Source: CAD feature listing. Evaluate the final solid. Frame: model axes, mm. A direction names the side the tool comes from. Round coordinates to 2 decimals unless told otherwise and drop trailing zeros. Order: outer loops, then holes, each group sorted by start corner. A loop starts at its lowest first (then second) coordinate and runs counter-clockwise, first axis right, second up. Notation, with made-up numbers: (-17, 53.5) -> (36, 53.5) arc R29 cw to (36, 79.5) -> close; hole circle Ø10 at (39, 8). An arc over 180 degrees is marked (long way). Answer as CSV lines item,"result".
from build123d import *

# Parameters (mm, degrees)
SKETCH_1_W           = 2
SKETCH_1_H           = 2
EXTRUDE_1_DEPTH      = 3
EXTRUDE_2_DEPTH      = 3.25
EXTRUDE_2_DEPTH_BACK = 5.25
SKETCH_2_R           = 1.35
EXTRUDE_5_DEPTH      = 1
EXTRUDE_START        = -1
EXTRUDE_6_DEPTH      = 1
EXTRUDE_7_DEPTH      = 10
EXTRUDE_7_DEPTH_BACK = 10


with BuildPart() as part:
    # 草图1 → 凸台-拉伸1 (new body)
    with BuildSketch(Plane.XY):
        Rectangle(SKETCH_1_W, SKETCH_1_H)
    extrude(amount=EXTRUDE_1_DEPTH)

    # 草图2 → 凸台-拉伸2 (add, two sides: drawn at the far end of the back side and taken through both)
    with BuildSketch(Plane(origin=(0, 1, 0), x_dir=(1, 0, 0), z_dir=(0, 1, 0)).offset(-EXTRUDE_2_DEPTH_BACK)):
        with Locations(Location((0, -4, 0), (0, 0, 270))):
            Circle(SKETCH_2_R)
    extrude(amount=EXTRUDE_2_DEPTH + EXTRUDE_2_DEPTH_BACK)

    # 草图6 → 凸台-拉伸5 (add)
    with BuildSketch(Plane(origin=(0, -2.75, 0), x_dir=(-1, 0, 0), z_dir=(0, -1, 0))):
        with BuildLine():
            Line((-1.75, -4), (1.75, -4))
            ThreePointArc((1.75, -4), (0, -2.25), (-1.75, -4))
        make_face()
    extrude(amount=-EXTRUDE_5_DEPTH)

    # 草图7 → 凸台-拉伸6 (add)
    with BuildSketch(Plane(origin=(0, 2.75, 0), x_dir=(1, 0, 0), z_dir=(0, 1, 0)).offset(EXTRUDE_START)):
        with BuildLine():
            Line((1.75, -4), (-1.75, -4))
            ThreePointArc((-1.75, -4), (0, -2.25), (1.75, -4))
        make_face()
    extrude(amount=EXTRUDE_6_DEPTH)

    # 草图12 → 凸台-拉伸7 (add, two sides: drawn at the far end of the back side and taken through both)
    with BuildSketch(Plane(origin=(0, 0, 0), x_dir=(1, 0, 0), z_dir=(0, 1, 0)).offset(-EXTRUDE_7_DEPTH_BACK)):
        Polygon((10, 0), (-10, 0), (-14, 6.92820323), (-12.267949192, 7.92820323), (-8.845299462, 2), (8.845299462, 2), (12.267949192, 7.92820323), (14, 6.92820323), align=None)
    extrude(amount=EXTRUDE_7_DEPTH + EXTRUDE_7_DEPTH_BACK)


solid = part.part
1. Section query B-B on x = 0. Return loops of the section in (y, z).
Results below:
outline,"(-10, -2) -> (10, -2) -> (10, 0) -> (1, 0) -> (1, 2.65) -> (1.75, 2.65) -> (1.75, 2.25) -> (2.75, 2.25) -> (2.75, 2.65) -> (4.25, 2.65) -> (4.25, 5.35) -> (-4.25, 5.35) -> (-4.25, 2.65) -> (-2.75, 2.65) -> (-2.75, 2.25) -> (-1.75, 2.25) -> (-1.75, 2.65) -> (-1, 2.65) -> (-1, 0) -> (-10, 0) -> close"
2. Reachability of faces 1 (the flat face through (-0.3, 2.75, 2.5)), 2 (the flat face through (-0.3, 1.75, 2.5)), 3 (the flat face through (0, -4.25, 4)), 4 (the flat face through (-10.581, -0.14, -5.006)) from +Z, -Z, +X, -X, +Y, -Y: full face, straight path, thin tool, end or side. Return the list, or none.
Results below:
face 1,"+Y"
face 2,"none"
face 3,"+Z, +X, -X, -Y"
face 4,"-Z, +Y, -Y"
3. Mould query, pull axis Y, two halves, no side actions, for faces 5 (the flat face through (10.53, -0.14, -4.92)), 6 (the flat face through (0, 4.25, 4)), 7 (the cylindrical face through (0.406, -0.059, 5.288)). Classes: released by +Y, released by -Y, zero draft, split by the parting line, or undercut.
Results below:
face 5,"zero draft"
face 6,"released by +Y"
face 7,"undercut"
4. Section query A-A on z = -2.75. Return loops of the section in (x, y).
Results below:
outline,"(-11.59, -10) -> (-9.28, -10) -> (-9.28, 10) -> (-11.59, 10) -> close; (9.28, -10) -> (11.59, -10) -> (11.59, 10) -> (9.28, 10) -> close"
5. Pin query (flat end, axial travel): pin 1 (1.5 mm diameter, centred on y = 2.5, z = 0.5, fed in from +X); pin 2 (0.5 mm diameter, centred on x = 0, z = 3, fed in from -Y); pin 3 (1 mm diameter, centred on y = 0, z = 1.5, fed in from -X). Return the tip coordinate at first contact, or that it passes through.
Results below:
pin 1,"x = 10.14"
pin 2,"y = -4.25"
pin 3,"x = -1"
6. Line query: L1, parallel to Z at x = 4.75, y = 6.25; L2, parallel to X at y = -6, z = -2.5; L3, parallel to X at y = -2.5, z = -6.5. Output: solid intervals per line, ascending. Write a range as [from, to].
Results below:
L1,"[-2, 0]"
L2,"[-11.44, -9.13], [9.13, 11.44]"
L3,"[-13.75, -11.44], [11.44, 13.75]"
